from build123d import *

# Parameters (mm, degrees)
SKETCH5_W           = 6.1595
SKETCH5_H           = 101.6
SKETCH5_W_2         = 101.6
SKETCH5_H_2         = 6.1595
BOSS_EXTRUDE1_DEPTH = 19.05
SKETCH6_W           = 333.025633445
SKETCH6_H           = 150.821732437
CUT_EXTRUDE1_DEPTH  = 205.486
SKETCH7_W           = 172.839732196
SKETCH7_H           = 155.996881263
CUT_EXTRUDE2_DEPTH  = 205.486


with BuildPart() as part:
    # Sketch2 → Loft1 section 0
    with BuildSketch(Plane(origin=(0, 127, 0), x_dir=(1, 0, 0), z_dir=(0, 1, 0))):
        with BuildLine():
            Line((-50.8, -50.8), (278.13, -50.8))
            Line((278.13, -50.8), (278.13, 276.352))
            Line((278.13, 276.352), (-50.8, 276.352))
            Line((-50.8, 276.352), (-50.8, -50.8))
        make_face()
    # Sketch1 → Loft1 section 1
    with BuildSketch(Plane(origin=(0, 0, 0), x_dir=(1, 0, 0), z_dir=(0, 1, 0))):
        with BuildLine():
            Line((0, 0), (227.33, 0))
            Line((227.33, 0), (227.33, 225.552))
            Line((227.33, 225.552), (0, 225.552))
            Line((0, 225.552), (0, 0))
        make_face()
    loft()

    # Sketch4 → Cut-Loft3 section 0
    with BuildSketch(Plane.XZ):
        with BuildLine():
            Line((208.28, -19.05), (19.05, -19.05))
            Line((19.05, -19.05), (19.05, -206.502))
            Line((19.05, -206.502), (208.28, -206.502))
            Line((208.28, -206.502), (208.28, -19.05))
        make_face()
    # Sketch3 → Cut-Loft3 section 1
    with BuildSketch(Plane(origin=(0, 127, 0), x_dir=(1, 0, 0), z_dir=(0, 1, 0))):
        with BuildLine():
            Line((-31.75, 257.302), (-31.75, -31.75))
            Line((-31.75, -31.75), (259.08, -31.75))
            Line((259.08, -31.75), (259.08, 257.302))
            Line((259.08, 257.302), (-31.75, 257.302))
        make_face()
    loft(mode=Mode.SUBTRACT)

    # Sketch5 → Boss-Extrude1 (add)
    with BuildSketch(Plane.XZ):
        with Locations((3.07975, -112.776)):
            Rectangle(SKETCH5_W, SKETCH5_H)
        with Locations((15.97025, -112.776)):
            Rectangle(SKETCH5_W, SKETCH5_H)
        with Locations((113.665, -3.07975)):
            Rectangle(SKETCH5_W_2, SKETCH5_H_2)
        with Locations((113.665, -15.97025)):
            Rectangle(SKETCH5_W_2, SKETCH5_H_2)
        with Locations((223.36125, -113.665)):
            Rectangle(SKETCH5_W, SKETCH5_H)
        with Locations((210.47075, -113.665)):
            Rectangle(SKETCH5_W, SKETCH5_H)
        with Locations((112.776, -223.36125)):
            Rectangle(SKETCH5_W_2, SKETCH5_H_2)
        with Locations((112.776, -210.47075)):
            Rectangle(SKETCH5_W_2, SKETCH5_H_2)
    extrude(amount=BOSS_EXTRUDE1_DEPTH)

    # Sketch6 → Cut-Extrude1 (cut)
    with BuildSketch(Plane.XY.offset(-113.2205)):
        with Locations((111.617183278, 51.589133782)):
            Rectangle(SKETCH6_W, SKETCH6_H)
    extrude(amount=-CUT_EXTRUDE1_DEPTH, mode=Mode.SUBTRACT)

    # Sketch7 → Cut-Extrude2 (cut)
    with BuildSketch(Plane.ZY.offset(-113.2205)):
        with Locations((-29.906934154, 52.245596061)):
            Rectangle(SKETCH7_W, SKETCH7_H)
    extrude(amount=-CUT_EXTRUDE2_DEPTH, mode=Mode.SUBTRACT)


solid = part.part
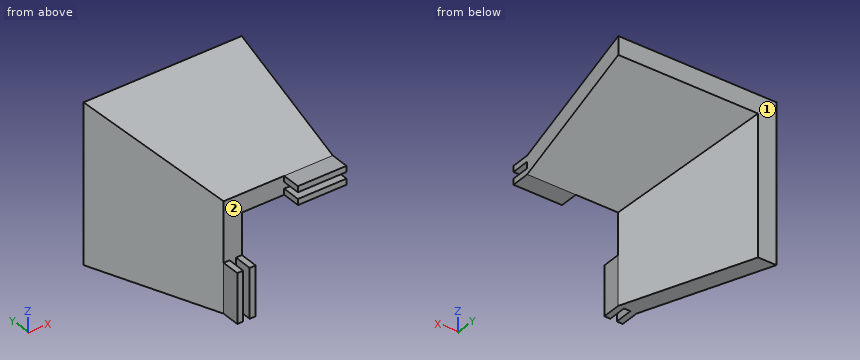
The model under review builds one solid part; all positions refer to its coordinate system, in mm. Face numbers are marked on the shaded views. Round coordinates to 2 decimals unless told otherwise and drop trailing zeros. Return JSON: item names as keys, results as strings.
(1) The part is to be moulded in two halves that separate along X. For the marked faces 1 and 2, say which applies: released by +X, released by -X, zero draft, split by the parting line, or undercut.
Solved:
{"face 1": "zero draft", "face 2": "undercut"}
(2) For line 1 (X direction, y = -9, z = -71); line 2 (Z direction, x = 10.5, y = 9); line 3 (X direction, y = 37, z = -86), list the stretches that pass through material, from the lowest coordinate up.
Solved:
{"line 1": "0 to 6.16, 12.89 to 19.05", "line 2": "-113.22 to 3.6", "line 3": "-14.8 to 4.25"}
(3) For pin 1 (2 mm diameter, centred on x = 84.5, y = 6.5, fed in from +Z); pin 2 (6 mm diameter, centred on x = 9, y = 88, fed in from +Z); pin 3 (9.5 mm diameter, centred on x = 95.5, y = -5.5, fed in from -Z), all flat-tipped, find the tip position at first contact; note any pin that passes through.
Solved:
{"pin 1": "z = 3", "pin 2": "z = 36.4", "pin 3": "z = -19.05"}
(4) Add section A-A on y = -5. State how many separate pieces and enclosed holes the cut face has, plus the area to 3 significant figures.
Solved:
{"separate pieces": "4", "enclosed holes": "0", "area": "1,250 mm2"}
